Source: CAD feature listing. Evaluate the final solid. Frame: model axes, mm. A direction names the side the tool comes from. Round coordinates to 2 decimals unless told otherwise and drop trailing zeros. Order: outer loops, then holes, each group sorted by start corner. A loop starts at its lowest first (then second) coordinate and runs counter-clockwise, first axis right, second up. Notation, with made-up numbers: M 68.5,81 L 115.5,81 A26 cw 115.5,105 Z; hole C -8.5,63 d11. An arc over 180 degrees is marked long. Use one line per item in the form item = value. Start each with the question number.
Q1. Reachability of faces 4 (the cylindrical face through (36.79, -6.89, -7.04)), 5 (the flat face through (-36, -32, -27)), 6 (the flat face through (-1, -1.6, 0)) from +Z, -Z, +X, -X, +Y, -Y: full face, straight path, thin tool, end or side. Return the list, or none.
Q2. Section B-B (z = -15). Return the cut outline in (x, y), plus the area to 3 significant figures.
Q3. Pull-direction query (Z, two-part tool) for faces 1 (the cylindrical face through (-8.31, -0.81, -14.04)), 2 (the flat face through (0, -26, 21.6)), 3 (the flat face through (-37.6, -26, 0)); classes: pulls with the +Z half, pulls with the -Z half, needs draft (parallel to the pull), parting line crosses it, or undercut.
Q4. Section C-C (x = 20.5). Return the cut outline in (y, z), plus the area to 3 significant figures.
Q5. Material intervals for probe 1 along X at (y, z) = (-1, -15); probe 2 along X at (y, z) = (-6, 7); probe 3 along Y at (x, z) = (-33, 18), sorted ascending.
Q6. Contact query for flat-ended pins moving along their axis: pin 1 (12 mm diameter, centred on x = -8, z = -35.5, fed in from -Y); pin 2 (0.5 mm diameter, centred on y = -15.5, z = 21, fed in from +X); pin 3 (1.8 mm diameter, centred on y = -16, z = 21, fed in from -X). Output: stop coordinate, or through.
Q7. Section D-D (y = -38). Return the cut outline in (x, z).
Q8. Section A-A (x = 30.4). Return the cut outline in (y, z).
from build123d import *

# Parameters (mm, degrees)
F0_W      = 75.2
F0_H      = 43.2
F0_W_2    = 72
F0_H_2    = 40
F1_DEPTH  = 52
F2_R      = 2
F3_DEPTH  = 1.6
F5_DEPTH  = 36
F6_D      = 9
F8_D      = 2.8
F8_DEPTH  = 1.601
F9_D      = 5
F10_W     = 1
F10_H     = 20
F11_DEPTH = 25


with BuildPart() as f1:
    # F0 (on Front) → F1 (new body)
    with BuildSketch(Plane.XZ):
        Rectangle(F0_W, F0_H)
        Rectangle(F0_W_2, F0_H_2, mode=Mode.SUBTRACT)
    extrude(amount=F1_DEPTH)

    # F2
    f2_edges = [f1.edges().sort_by_distance(p)[0] for p in [
        (37.6, -26, 21.6),
        (-37.6, -26, 21.6),
        (-37.6, -26, -21.6),
        (37.6, -26, -21.6),
    ]]
    fillet(f2_edges, radius=F2_R)

    # F0 (on Front) → F3 (join)
    with BuildSketch(Plane.XZ):
        Rectangle(F0_W_2, F0_H_2)
    extrude(amount=F3_DEPTH)

    # F4 (on Right) → F5 (join, symmetric)
    with BuildSketch(Plane.YZ):
        Polygon((0, -21.6), (-52, -21.6), (-41.0421315348, -42.8069394041), align=None)
    extrude(amount=F5_DEPTH, both=True)

    # F6 (through all)
    with Locations(Plane(origin=(0, 0, 0), x_dir=(1, 0, 0), z_dir=(0, 1, 0))):
        with Locations((30.4, 6)):
            Hole(F6_D / 2)

    # F8 (through all, one way)
    with BuildSketch(Plane(origin=(36, 0, 0), x_dir=(0, -1, 0), z_dir=(-1, 0, 0))):
        with Locations((5.6, -6.5)):
            Circle(F8_D / 2)
    extrude(amount=-F8_DEPTH, mode=Mode.SUBTRACT)

    # F9 (through all)
    with Locations(Plane(origin=(0, 0, 0), x_dir=(1, 0, 0), z_dir=(0, 1, 0))):
        with Locations((-6, 15)):
            Hole(F9_D / 2)

    # F10 (on face) → F11 (cut)
    with BuildSketch(Plane.XY.offset(21.6)):
        with Locations((-32.2436588705, -14.5910207555)):
            Rectangle(F10_W, F10_H)
        with Locations((-28.8436588705, -14.5910207555)):
            Rectangle(F10_W, F10_H)
        with Locations((-25.4436588705, -14.5910207555)):
            Rectangle(F10_W, F10_H)
        with Locations((-22.0436588705, -14.5910207555)):
            Rectangle(F10_W, F10_H)
        with Locations((-18.6436588705, -14.5910207555)):
            Rectangle(F10_W, F10_H)
        with Locations((-15.2436588705, -14.5910207555)):
            Rectangle(F10_W, F10_H)
        with Locations((-11.8436588705, -14.5910207555)):
            Rectangle(F10_W, F10_H)
        with Locations((-8.4436588705, -14.5910207555)):
            Rectangle(F10_W, F10_H)
        with Locations((-5.0436588705, -14.5910207555)):
            Rectangle(F10_W, F10_H)
        with Locations((1.7563411295, -14.5910207555)):
            Rectangle(F10_W, F10_H)
        with Locations((5.1563411295, -14.5910207555)):
            Rectangle(F10_W, F10_H)
        with Locations((-1.6436588705, -14.5910207555)):
            Rectangle(F10_W, F10_H)
        with Locations((8.5563411295, -14.5910207555)):
            Rectangle(F10_W, F10_H)
        with Locations((11.9563411295, -14.5910207555)):
            Rectangle(F10_W, F10_H)
        with Locations((15.3563411295, -14.5910207555)):
            Rectangle(F10_W, F10_H)
        with Locations((18.7563411295, -14.5910207555)):
            Rectangle(F10_W, F10_H)
        with Locations((22.1563411295, -14.5910207555)):
            Rectangle(F10_W, F10_H)
        with Locations((25.5563411295, -14.5910207555)):
            Rectangle(F10_W, F10_H)
        with Locations((28.9563411295, -14.5910207555)):
            Rectangle(F10_W, F10_H)
        with Locations((32.3563411295, -14.5910207555)):
            Rectangle(F10_W, F10_H)
    extrude(amount=-F11_DEPTH, mode=Mode.SUBTRACT)


solid = f1.part
Results list:
q1.face_4 = +X
q1.face_5 = -Z, -X, +Y, -Y
q1.face_6 = -Y
q2.outline = M -37.6,-52 L -36,-52 L -36,-1.6 L -8.5,-1.6 L -8.5,0 L -37.6,0 Z; M -3.5,-1.6 L 36,-1.6 L 36,-52 L 37.6,-52 L 37.6,0 L -3.5,0 Z
q2.area = 274 mm2
q3.face_1 = undercut
q3.face_2 = pulls with the +Z half
q3.face_3 = needs draft
q4.outline = M -52,-21.6 L -41.04,-42.81 L 0,-21.6 L 0,21.6 L -52,21.6 L -52,20 L -1.6,20 L -1.6,-20 L -52,-20 Z
q4.area = 782 mm2
q5.probe_1 = -37.6 to -8.5, -3.5 to 37.6
q5.probe_2 = -37.6 to -36, 36 to 37.6
q5.probe_3 = -1.6 to 0
q6.pin_1 = -47.92
q6.pin_2 = 37.24
q6.pin_3 = -37.54
q7.outline = M -37.6,-19.6 A2 ccw -35.6,-21.6 L -36,-21.6 L -36,-41.24 L 36,-41.24 L 36,-21.6 L 35.6,-21.6 A2 ccw 37.6,-19.6 L 37.6,19.6 A2 ccw 35.6,21.6 L -35.6,21.6 A2 ccw -37.6,19.6 Z; hole M -36,-20 L 36,-20 L 36,20 L -36,20 Z
q8.outline = M -52,-21.6 L -41.04,-42.81 L 0,-21.6 L 0,-10.5 L -1.6,-10.5 L -1.6,-20 L -52,-20 Z; M -52,20 L -1.6,20 L -1.6,-1.5 L 0,-1.5 L 0,21.6 L -52,21.6 Z
